Verification items for the finished model (mm, model axes). A direction names the side the tool comes from. Give positions to 0.01 mm unless a question says otherwise; leave off trailing zeros. Loops run counter-clockwise (first coordinate to the right, second up) from the corner with the lowest first, then second, coordinate; pieces in that order, holes last. Notation, with made-up numbers: M 84.5,-4 L 120.5,-4 A13 ccw 120.5,17 Z; hole C 57.5,-8 d8. An arc over 180 degrees is marked long. Put each result on its own line as item: value. Start each with the question number.
Autodesk Inventor part; units mm, degrees
ref_plane "YZ Plane" through (0, 0, 0) normal (1, 0, 0) x (0, 1, 0)
ref_plane "XZ Plane" through (0, 0, 0) normal (0, 1, 0) x (-1, 0, 0)
ref_plane "XY Plane" through (0, 0, 0) normal (0, 0, 1) x (1, 0, 0)
sketch "スケッチ1" plane through (0, 0, 0) normal (0, 0, 1) x (1, 0, 0)
  line L0 (0, 0) -> (60, 0)
  line L1 (60, 0) -> (60, 60)
  line L2 (60, 60) -> (0, 60)
  line L3 (0, 60) -> (0, 0)
  dimension "d0" = 60
  dimension "d1" = 60
extrude "押し出し1" add sketch "スケッチ1" along normal blind 30
sketch "スケッチ2" plane through (0, 0, 30) normal (0, 0, 1) x (1, 0, 0)
  line L0 (60, 0) -> (60, 60)
  line L1 (60, 60) -> (0, 60)
  point P0 (0, 0)
  point P1 (22, 49.5)
  point P2 (37, 49.5)
  point P3 (52.5, 34)
  point P4 (52.5, 19)
  dimension "d4" = 7.5
  dimension "d5" = 7.5
  dimension "d6" = 10.5
  dimension "d7" = 10.5
  dimension "d8" = 15
  dimension "d9" = 15
  dimension "d10" = 23
  dimension "d11" = 26
hole "穴1" at (22, 49.5, 30) at (37, 49.5, 30) at (52.5, 34, 30) at (52.5, 19, 30) direction (0, 0, -1) diameter 5 end through all
sketch "スケッチ3" plane through (0, 0, 30) normal (0, 0, 1) x (1, 0, 0)
  line L0 (22, 49.5) -> (37, 49.5)
  circle A0 centre (52.5, 34) radius 2.5
  line L1 (37, 49.5) -> (52.5, 34)
  line L2 (52.5, 34) -> (52.5, 19)
  line L3 (22, 49.5) -> (22, 19)
  line L4 (22, 19) -> (52.5, 19)
  line L5 (60, 37.1066) -> (40.1066, 57)
  line L6 (40.1066, 57) -> (14.5, 57)
  line L7 (14.5, 57) -> (14.5, 11.5)
  line L8 (14.5, 11.5) -> (60, 11.5)
  line L9 (60, 11.5) -> (60, 37.1066)
  line L10 (14.5, 57) -> (44.5, 57)
  line L11 (44.5, 57) -> (44.5, 42)
  line L12 (44.5, 42) -> (14.5, 42)
  line L13 (14.5, 42) -> (14.5, 57)
  line L14 (60, 11.5) -> (45, 11.5)
  line L15 (45, 11.5) -> (45, 41.5)
  line L16 (45, 41.5) -> (60, 41.5)
  line L17 (60, 41.5) -> (60, 11.5)
  circle A1 centre (52.5, 19) radius 2.5
  circle A2 centre (52.5, 34) radius 2.5
  circle A3 centre (37, 49.5) radius 2.5
  circle A4 centre (22, 49.5) radius 2.5
  line L18 (60, 0) -> (60, 60)
  line L19 (60, 60) -> (0, 60)
  line L20 (0, 60) -> (0, 0)
  line L21 (0, 0) -> (60, 0)
  line L22 (14.5, 42) -> (45, 11.5)
  line L23 (24.0029, 51.8905) -> (54.5029, 21.3905)
  line L24 (38.7868, 57) -> (60, 35.7868)
  point P0 (52.5, 26.5)
  point P1 (45, 19)
  point P2 (22, 42)
  point P3 (39.2529, 36.6405)
  point P4 (45, 30.8934)
  point P5 (33.8934, 42)
  dimension "d19" = 7.5
  dimension "d20" = 7.5
  dimension "d21" = 7.5
  dimension "d22" = 30
  dimension "d23" = 30
  dimension "d50" = 7.5
  dimension "d52" = 30
extrude "押し出し2" cut sketch "スケッチ3" against normal blind 30 contours L12 L23 L15 L4 L22 L3 | L3 L22 L12 | L22 L4 L3 | L3 L4 L22 L8 L7 | L7 L8 L18 L21 L20 L19 L16 L5 L11 L10 L6 | L4 L15 L22 | L24 L6 L5 L11 | L11 L5 L16 L24 | L16 L5 L9 L24 | L5 L10 L11 | L16 L17 L5
sketch "スケッチ15" plane through (60, 35.7868, 0) normal (0.7071068, 0.7071068, 0) x (-0.7071068, 0.7071068, 0)
  line L0 (0, 30) -> (30, 30)
  line L1 (0, 0) -> (0, 30)
  line L2 (30, 0) -> (0, 0)
  line L3 (30, 30) -> (30, 0)
  point P0 (17.1213, 0)
extrude "押し出し11" add sketch "スケッチ15" along normal blind 30
sketch "スケッチ16" plane through (60, 35.7868, 30) normal (0.7071068, -0.7071068, 0) x (-0.7071068, -0.7071068, 0)
  line L0 (0, 30) -> (0, 0)
  line L1 (0, 30) -> (-30, 30)
  line L2 (-30, 0) -> (-30, 30)
  line L3 (0, 0) -> (-30, 0)
  line L4 (0, 0) -> (-30, 30)
  point P0 (67.7315, 30)
extrude "押し出し12" cut sketch "スケッチ16" against normal blind 30 contours L3 L2 L4
sketch "スケッチ18" plane through (60, 35.7868, 30) normal (0.5, 0.5, 0.7071068) x (0.7071068, -0.7071068, 0)
  line L0 (0, 42.4264) -> (0, 0)
  line L1 (0, 42.4264) -> (-30, 42.4264)
  line L2 (-30, 0) -> (-30, 42.4264)
  line L3 (0, 0) -> (-30, 0)
  point P0 (-17.1213, -26.6802)
extrude "押し出し13" add sketch "スケッチ18" along normal blind 30
sketch "スケッチ19" plane through (81.2132, 57, 0) normal (0.5, 0.5, -0.7071068) x (-0.5, -0.5, -0.7071068)
  line L0 (21.2132, 0) -> (0, 0)
  line L1 (0, 30) -> (-30, 30)
  line L2 (0, 0) -> (-30, 30)
  line L3 (-30, 30) -> (0, 30)
  line L4 (0, 0) -> (-30, 0)
  line L5 (0, 30) -> (-30, 0)
  line L6 (0, 0) -> (0, 30)
  line L7 (0, 30) -> (-30, 30)
  line L8 (-30, 0) -> (-30, 30)
  line L9 (0, 0) -> (-30, 0)
  point P0 (69.1066, 17.1213)
  point P1 (-15, 15)
extrude "押し出し14" cut sketch "スケッチ19" against normal through all contours L5 L2 L1 | L2 L5 L8 | L2 L4 L5
sketch "スケッチ20" plane through (0, 0, 30) normal (0, 0, 1) x (1, 0, 0)
  circle A0 centre (52.5, 19) radius 2.5
  circle A1 centre (52.5, 34) radius 2.5
  circle A2 centre (37, 49.5) radius 2.5
  circle A3 centre (22, 49.5) radius 2.5
  line L0 (60, 35.7868) -> (38.7868, 57)
  line L1 (38.7868, 57) -> (14.5, 57)
  line L2 (14.5, 57) -> (14.5, 42)
  line L3 (14.5, 42) -> (33.8934, 42)
  line L4 (33.8934, 42) -> (45, 30.8934)
  line L5 (45, 30.8934) -> (45, 11.5)
  line L6 (45, 11.5) -> (60, 11.5)
  line L7 (60, 11.5) -> (60, 35.7868)
  line L8 (38.7868, 57) -> (60, 78.2132)
  line L9 (38.7868, 57) -> (60, 78.2132)
  line L10 (60, 78.2132) -> (81.2132, 57)
  line L11 (81.2132, 57) -> (60, 35.7868)
  point P0 (0, 0)
extrude "押し出し15" cut sketch "スケッチ20" along normal blind 15 contours L0 L8 L10 L11
sketch "スケッチ23" plane through (81.2132, 57, 0) normal (0.8535534, -0.1464466, 0.5) x (0.5, 0.5, -0.7071068)
  line L0 (0, 21.2132) -> (0, 0)
  line L1 (-27.4264, 21.2132) -> (-42.4264, 0)
  line L2 (0, 0) -> (-27.4264, 0)
  line L3 (-27.4264, 0) -> (-27.4264, 21.2132)
  line L4 (-27.4264, 21.2132) -> (0, 21.2132)
  line L5 (0, 21.2132) -> (0, 0)
  point P0 (-69.1066, -36.7591)
  point P1 (-17.4264, 12.4132)
  point P2 (-7.4264, 12.4132)
  dimension "d71" = 10
  dimension "d72" = 10
  dimension "d93" = 8.8
  dimension "d94" = 8.8
hole "穴2" at (70.6821, 58.8821, 18.5289) at (75.6821, 63.8821, 11.4579) direction (-0.8535534, 0.1464466, -0.5) diameter 5 depth 8
sketch "スケッチ24" plane through (60, 78.2132, 0) normal (-0.1464466, 0.8535534, 0.5) x (0.8535534, -0.1464466, 0.5)
  line L0 (21.2132, -27.4264) -> (21.2132, -42.4264)
  line L1 (-15, -21.2132) -> (0, 0)
  line L2 (21.2132, -27.4264) -> (0, -27.4264)
  line L3 (0, -27.4264) -> (0, 0)
  line L4 (0, 0) -> (21.2132, 0)
  line L5 (21.2132, 0) -> (21.2132, -27.4264)
  point P0 (-39.7591, -69.1066)
  point P1 (12.4132, -17.4264)
  point P2 (12.4132, -7.4264)
  dimension "d82" = 10
  dimension "d83" = 10
  dimension "d95" = 8.8
  dimension "d96" = 8.8
hole "穴3" at (61.8821, 67.6821, 18.5289) at (66.8821, 72.6821, 11.4579) direction (0.1464466, -0.8535534, -0.5) diameter 5 depth 8
equation "\"d20\" = d19"
equation "\"d23\" = d22"
properties part number "EX-L-Connect"
Q1. Cross-section at D-D, the plane x = 37. Record the boundary of the cut face in (y, z), then the cut area to 3 significant figures.
Q2. Set-up check for faces 4 (the face through (63.835, 59.56, 14.415)), 5 (the face through (27, 57, 15)), 6 (the face through (45, 21, 15)): record each of +Z, -Z, +X, -X, +Y, -Y from which the full face is reachable in a straight line by a thin tool's end or side.
Q3. Cross-section at A-A, the plane x = 52.5. Record the boundary of the cut face in (y, z), then the cut area to 3 significant figures.
Q4. Cross-section at C-C, the plane y = 19. Record the boundary of the cut face in (x, z).
Q5. Scan lines: L1, parallel to X at y = 49.5, z = 18.75; L2, parallel to X at y = 19, z = 10.25; L3, parallel to X at y = 49, z = 11. Record each from-to range of solid material in increasing order.
Q6. Go/stop test with flat-tipped pins: pin 1 (3 mm diameter, centred on x = 52.5, y = 19, fed in from +Z); pin 2 (1.5 mm diameter, centred on y = 48.5, z = 4, fed in from +X); pin 3 (10 mm diameter, centred on x = 33, z = 8, fed in from -Y); pin 4 (9.5 mm diameter, centred on y = 21.5, z = 11, fed in from -X). Record where each tip stops, or that it passes through.
Q7. Release check for a two-part mould opening along Z. For faces 1 (the face through (71.926, 55.814, 15.507)), 2 (the face through (66.556, 42.343, 8.852)), 3 (the face through (67.72, 57.49, 15.07)) record: pulls with the +Z half, pulls with the -Z half, needs draft (parallel to the pull), parting line crosses it, or undercut.
Q8. Cross-section at B-B, the plane y = 49.5. Record the boundary of the cut face in (x, z).
Ans:
1. outline: M 38.89,0 L 47,0 L 47,30 L 38.89,30 Z; M 52,0 L 57,0 L 57,30 L 52,30 Z
1. area: 393 mm^2
2. face 4: none
2. face 5: +Z, -Z, -X, +Y
2. face 6: +Z, -Z, -X, -Y
3. outline: M 11.5,0 L 16.5,0 L 16.5,30 L 11.5,30 Z; M 21.5,0 L 31.5,0 L 31.5,30 L 21.5,30 Z; M 36.5,0 L 70.71,0 L 70.71,10.61 L 59.35,30 L 36.5,30 Z
3. area: 1,370 mm^2
4. outline: M 45,0 L 50,0 L 50,30 L 45,30 Z; M 55,0 L 60,0 L 60,30 L 55,30 Z
5. L1: x = 14.5 to 19.5, 24.5 to 34.5, 39.5 to 68.94
5. L2: x = 45 to 50, 55 to 60
5. L3: x = 14.5 to 19.55, 24.45 to 34.55, 39.45 to 73.21
6. pin 1: passes through
6. pin 2: stops at x = 73.46
6. pin 3: stops at y = 37.89
6. pin 4: stops at x = 45
7. face 1: pulls with the +Z half
7. face 2: needs draft
7. face 3: undercut
8. outline: M 14.5,0 L 19.5,0 L 19.5,30 L 14.5,30 Z; M 24.5,0 L 34.5,0 L 34.5,30 L 24.5,30 Z; M 39.5,0 L 73.71,0 L 73.71,10.61 L 62.35,30 L 39.5,30 Z
